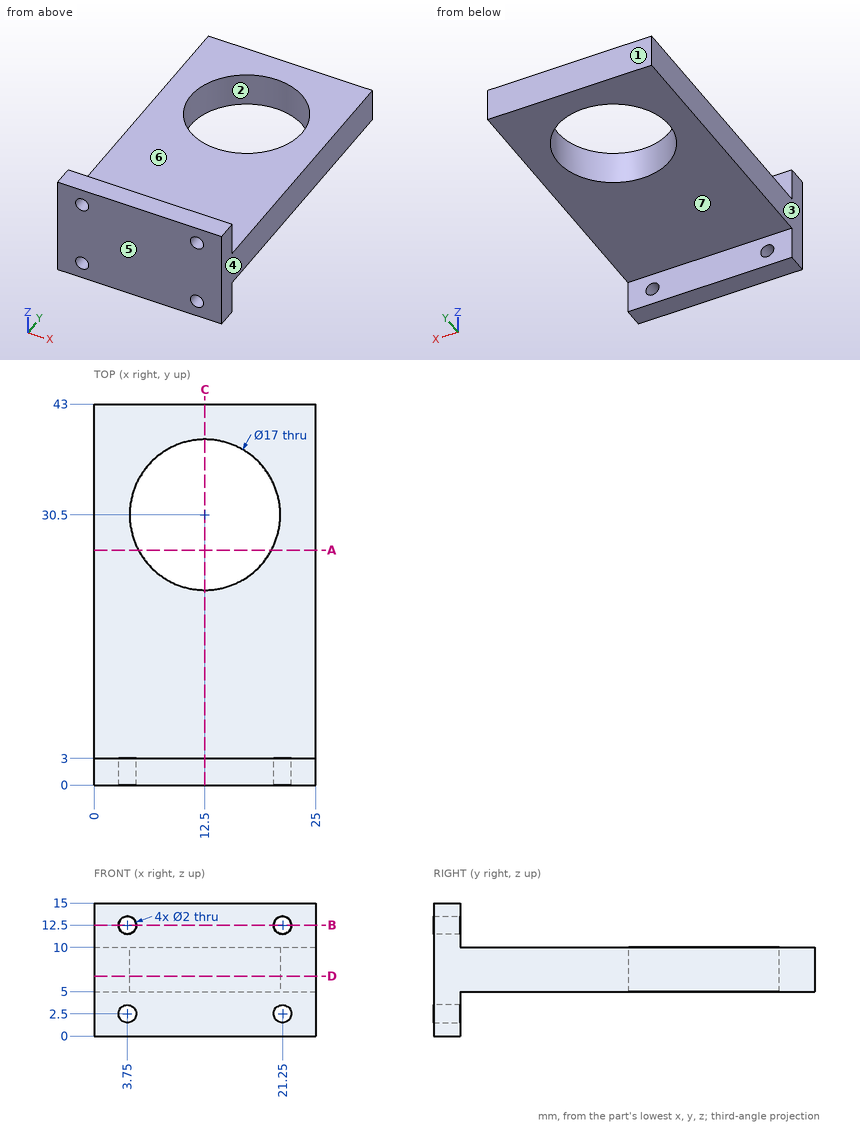
Geometry check sheet. Reference: drawing and pictorial views, mm from the part's lowest x, y, z. A direction names the side the tool comes from. Give positions to 0.01 mm unless a question says otherwise; leave off trailing zeros. Loops run counter-clockwise (first coordinate to the right, second up) from the corner with the lowest first, then second, coordinate; pieces in that order, holes last. Notation, with made-up numbers: (-27, -7) - (8, -7) arc R4 ccw to (8, -2) - close; hole circle Ø4 at (-5, -11). An arc over 180 degrees is marked (long way). One line per question, with ' | ' between items. Start each with the question number.
1. Cross-section at D-D, the plane z = 6.75. Enter the section's corners in (x, y), plus the area to 3 significant figures.
2. Gauge pin test, flat ends, axial feed: pin 1 Ø4 at (x, z) = (12, 2) entering from +Y; pin 2 Ø7.5 at (x, y) = (15, 21) entering from +Z; pin 3 Ø7.5 at (x, y) = (11.5, 20.5) entering from -Z. Record the tip position at first contact, or that the pin passes through.
3. Material ranges on line 1 along X through (y, z) = (0.7, 12.5); line 2 along Z through (x, y) = (7, 7); line 3 along Y through (x, z) = (10, 4.5), recorded low to high. Write a range as [from, to].
4. Cross-section at C-C, the plane x = 12.5. Enter the section's corners in (y, z), plus the area to 3 significant figures.
5. Set-up check for the marked faces 5, 6 and 7: record each of +Z, -Z, +X, -X, +Y, -Y from which the full face is reachable in a straight line by a thin tool's end or side.
6. Cross-section at A-A, the plane y = 26.5. Enter the section's corners in (x, z).
7. Draft check along X on the marked faces 1, 2, 3 and 4. Enter one of: released by +X, released by -X, zero draft, split by the parting line, or undercut.
8. Cross-section at B-B, the plane z = 12.5. Enter the section's corners in (x, y).
Check result:
1) outline: (0, 0) - (25, 0) - (25, 43) - (0, 43) - close; hole circle Ø17 at (12.5, 30.5) | area: 848 mm2
2) pin 1: stops at y = 3 | pin 2: stops at z = 10 | pin 3: stops at z = 5
3) line 1: x = [0, 2.75], [4.75, 20.25], [22.25, 25] | line 2: z = [5, 10] | line 3: y = [0, 3]
4) outline: (0, 0) - (3, 0) - (3, 5) - (22, 5) - (22, 10) - (3, 10) - (3, 15) - (0, 15) - close; (39, 5) - (43, 5) - (43, 10) - (39, 10) - close | area: 160 mm2
5) face 5: +Z, -Z, +X, -X, -Y | face 6: +Z, +X, -X, +Y | face 7: -Z, +X, -X, +Y
6) outline: (0, 5) - (5, 5) - (5, 10) - (0, 10) - close; (20, 5) - (25, 5) - (25, 10) - (20, 10) - close
7) face 1: zero draft | face 2: undercut | face 3: released by -X | face 4: released by +X
8) outline: (0, 0) - (2.75, 0) - (2.75, 3) - (0, 3) - close; (4.75, 0) - (20.25, 0) - (20.25, 3) - (4.75, 3) - close; (22.25, 0) - (25, 0) - (25, 3) - (22.25, 3) - close
